from build123d import *

# Parameters (mm, degrees)
F0_W     = 63.5
F0_H     = 44.45
F1_DEPTH = 588.9625
F3_DEPTH = 25.4
F2_W     = 7.9375
F2_H     = 425.45
F4_DEPTH = 9.525
F6_DEPTH = 9.525
F5_W     = 9.525
F5_H     = 20.7645
F5_H_2   = 28.575
F7_DEPTH = 44.451
F8_SIZE  = 11.90625


with BuildPart() as f1:
    # F0 (on Top) → F1 (new body)
    with BuildSketch(Plane.XY):
        with Locations((31.75, 22.225)):
            Rectangle(F0_W, F0_H)
    extrude(amount=F1_DEPTH)

    # F2 (on face) → F3 (cut)
    with BuildSketch(Plane.YZ.offset(63.5)):
        Polygon((26.9875, 579.4375), (17.4625, 579.4375), (17.4625, 522.2875), (18.25625, 522.2875), (26.19375, 522.2875), (26.9875, 522.2875), align=None)
        Polygon((26.19375, 96.8375), (18.25625, 96.8375), (17.4625, 96.8375), (17.4625, 26.9875), (26.9875, 26.9875), (26.9875, 96.8375), align=None)
    extrude(amount=-F3_DEPTH, mode=Mode.SUBTRACT)

    # F2 (on face) → F4 (cut)
    with BuildSketch(Plane.YZ.offset(63.5)):
        with Locations((22.225, 309.5625)):
            Rectangle(F2_W, F2_H)
    extrude(amount=-F4_DEPTH, mode=Mode.SUBTRACT)

    # F5 (on face) → F6 (cut)
    with BuildSketch(Plane.XZ):
        Polygon((35.71875, 522.0335), (28.575, 522.0335), (27.78125, 522.0335), (27.78125, 96.8375), (35.71875, 96.8375), align=None)
    extrude(amount=-F6_DEPTH, mode=Mode.SUBTRACT)

    # F5 (on face) → F7 (cut, through all)
    with BuildSketch(Plane.XZ):
        with Locations((31.75, 569.05525)):
            Rectangle(F5_W, F5_H)
        Polygon((27.78125, 522.0335), (28.575, 522.0335), (35.71875, 522.0335), (36.5125, 522.0335), (36.5125, 542.798), (26.9875, 542.798), (26.9875, 522.0335), align=None)
        Polygon((35.71875, 96.8375), (27.78125, 96.8375), (26.9875, 96.8375), (26.9875, 68.2625), (36.5125, 68.2625), (36.5125, 96.8375), align=None)
        with Locations((31.75, 41.275)):
            Rectangle(F5_W, F5_H_2)
    extrude(amount=-F7_DEPTH, mode=Mode.SUBTRACT)

    # F8
    f8_edges = [f1.edges().sort_by_distance(p)[0] for p in [
        (63.5, 44.45, 294.48125),
        (0, 44.45, 294.48125),
        (63.5, 0, 294.48125),
    ]]
    chamfer(f8_edges, length=F8_SIZE)


solid = f1.part
Verification items for the finished model (mm, model axes). A direction names the side the tool comes from. Coordinates: 2 decimals unless noted, no trailing zeros. Order: outer loops, then holes, each group sorted by start corner. A loop starts at its lowest first (then second) coordinate and runs counter-clockwise, first axis right, second up. Notation, with made-up numbers: M 30,34 L 70,34 A23 ccw 70,67 Z; hole C 3,41 d2. An arc over 180 degrees is marked long. Return JSON: item names as keys, results as strings.
1) Cross-section at B-B, the plane z = 353. Record the boundary of the cut face in (x, y) (3 decimals).
Answer list:
{"outline": "M 0,0 L 27.781,0 L 27.781,9.525 L 35.719,9.525 L 35.719,0 L 51.594,0 L 63.5,11.906 L 63.5,18.256 L 53.975,18.256 L 53.975,26.194 L 63.5,26.194 L 63.5,32.544 L 51.594,44.45 L 11.906,44.45 L 0,32.544 Z"}
2) Access from +Z, -Z, +X, -X, +Y, -Y to the whole of each face (thin tool, end or side, straight path). Record for faces 5 (the flat face through (35.719, 5, 306)), 6 (the flat face through (26.988, 22, 41)), 7 (the flat face through (38.1, 22, 551)), 8 (the flat face through (31, 23, 0)).
Answer list:
{"face 5": "-Y", "face 6": "+Y, -Y", "face 7": "+X", "face 8": "-Z, +X, -X, +Y, -Y"}
3) Gauge pin test, flat ends, axial feed: pin 1 (3 mm diameter, centred on y = 3, z = 402.5, fed in from +X); pin 2 (5 mm diameter, centred on x = 60.5, z = 389, fed in from +Y); pin 3 (7.5 mm diameter, centred on x = 56.5, z = 401, fed in from -Y). Record the tip position at first contact, or that the pin passes through.
Answer list:
{"pin 1": "x = 56.09", "pin 2": "y = 38.04", "pin 3": "y = 1.16"}
4) Cross-section at A-A, the plane x = 46.5. Record the boundary of the cut face in (y, z).
Answer list:
{"outline": "M 0,0 L 44.45,0 L 44.45,588.96 L 0,588.96 Z; hole M 17.46,26.99 L 26.99,26.99 L 26.99,96.84 L 17.46,96.84 Z; hole M 17.46,522.29 L 26.99,522.29 L 26.99,579.44 L 17.46,579.44 Z"}
5) Release check for a two-part mould opening along X. For faces 1 (the flat face through (63.5, 27, 290)), 2 (the flat face through (32, 22, 579.438)), 3 (the flat face through (0, 16, 290)), 4 (the flat face through (59, 18.256, 307)) record: +X half, -X half, draft (parallel to the pull), parting line (faces both ways), or undercut.
Answer list:
{"face 1": "+X half", "face 2": "undercut", "face 3": "-X half", "face 4": "draft"}
6) Thickness scan on L1, parallel to Z at x = 36, y = 11; L2, parallel to Z at x = 51, y = 23; L3, parallel to X at y = 24, z = 405 (3 decimals). Record the ranges inside material, lowest first. Write a range as [from, to].
Answer list:
{"L1": "[0, 26.99], [55.56, 68.26], [96.84, 522.03], [542.8, 558.67], [579.44, 588.96]", "L2": "[0, 26.99], [96.84, 522.29], [579.44, 588.96]", "L3": "[0, 53.975]"}
